Source: CAD feature listing. Evaluate the final solid. Frame: model axes, mm. Face numbers are marked on the shaded views. A direction names the side the tool comes from. Round coordinates to 2 decimals unless told otherwise and drop trailing zeros. Loops run counter-clockwise (first coordinate to the right, second up) from the corner with the lowest first, then second, coordinate; pieces in that order, holes last. Notation, with made-up numbers: (61, 25.25) -> (101, 25.25) arc R24 ccw to (101, 36.25) -> close; hole circle Ø9 at (-26.75, -5). An arc over 180 degrees is marked (long way). Put each result on its own line as item: value. Start each with the question number.
1. Cut plane C-C (x = 3.5). Return the cut outline in (y, z) (1 decimal).
2. Set-up query: the marked faces 1 and 2. Return all of +Z, -Z, +X, -X, +Y, -Y with unobstructed straight access to the full face (end or side cutting, diameter ignored); none if empty.
3. Contact query for flat-ended pins moving along their axis: pin 1 (5 mm diameter, centred on y = 9, z = 25.5, fed in from +X); pin 2 (6.5 mm diameter, centred on y = 8, z = 102, fed in from -X); pin 3 (4 mm diameter, centred on x = 2.5, y = 9, fed in from +Z). Output: stop coordinate, or through.
4. Material intervals for L1, parallel to Y at x = 31.25, z = 58.42; L2, parallel to Z at x = 34, y = 11.75; L3, parallel to X at y = 12, z = 33, sorted ascending.
5. Cut plane A-A (z = 58.42). Return the cut outline in (x, y), then the cut area to 3 significant figures.
6. Cut plane B-B (y = 7.5). Return the cut outline in (x, z), then the cut area to 3 significant figures.
7. Cut plane D-D (y = 12.75). Return the cut outline in (x, z), then the cut area to 3 significant figures.
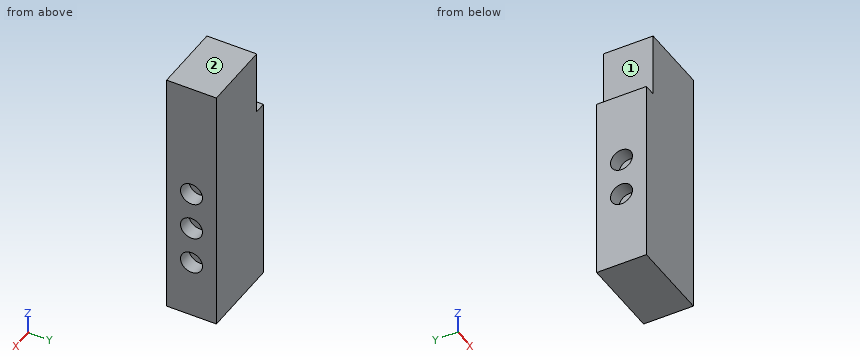
```python
from build123d import *

# Parameters (mm, degrees)
SKETCH1_W           = 35.56
SKETCH1_H           = 21.59
BOSS_EXTRUDE1_DEPTH = 81.28
SKETCH2_W           = 30.48
SKETCH2_H           = 21.59
BOSS_EXTRUDE2_DEPTH = 27.94
SKETCH3_R           = 4.7625
CUT_EXTRUDE1_DEPTH  = 6.35
SKETCH4_R           = 4.7625
CUT_EXTRUDE2_DEPTH  = 6.35


with BuildPart() as part:
    # Sketch1 → Boss-Extrude1 (new body)
    with BuildSketch(Plane.XY):
        with Locations((17.78, 10.795)):
            Rectangle(SKETCH1_W, SKETCH1_H)
    extrude(amount=BOSS_EXTRUDE1_DEPTH)

    # Sketch2 → Boss-Extrude2 (add)
    with BuildSketch(Plane.XY.offset(81.28)):
        with Locations((20.32, 10.795)):
            Rectangle(SKETCH2_W, SKETCH2_H)
    extrude(amount=BOSS_EXTRUDE2_DEPTH)

    # Sketch3 → Cut-Extrude1 (cut)
    with BuildSketch(Plane(origin=(35.56, 0, 0), x_dir=(0, 0, -1), z_dir=(1, 0, 0))):
        with Locations((-25.4, 10.795)):
            Circle(SKETCH3_R)
        with Locations((-41.91, 10.795)):
            Circle(SKETCH3_R)
        with Locations((-58.42, 10.795)):
            Circle(SKETCH3_R)
    extrude(amount=-CUT_EXTRUDE1_DEPTH, mode=Mode.SUBTRACT)

    # Sketch4 → Cut-Extrude2 (cut)
    with BuildSketch(Plane.ZY):
        with Locations((33.655, 10.795)):
            Circle(SKETCH4_R)
        with Locations((50.165, 10.795)):
            Circle(SKETCH4_R)
    extrude(amount=-CUT_EXTRUDE2_DEPTH, mode=Mode.SUBTRACT)


solid = part.part
```
Solution:
1. outline: (0, 0) -> (21.6, 0) -> (21.6, 81.3) -> (0, 81.3) -> close; hole circle Ø9.5 at (10.8, 33.7); hole circle Ø9.5 at (10.8, 50.2)
2. face 1: +Z, -X, +Y, -Y
2. face 2: +Z, +X, -X, +Y, -Y
3. pin 1: stops at x = 29.21
3. pin 2: stops at x = 5.08
3. pin 3: stops at z = 81.28
4. L1: y = 0 to 6.03, 15.56 to 21.59
4. L2: z = 0 to 20.73, 30.07 to 37.24, 46.58 to 53.75, 63.09 to 109.22
4. L3: x = 6.35 to 35.56
5. outline: (0, 0) -> (35.56, 0) -> (35.56, 6.03) -> (29.21, 6.03) -> (29.21, 15.56) -> (35.56, 15.56) -> (35.56, 21.59) -> (0, 21.59) -> close
5. area: 707 mm^2
6. outline: (0, 0) -> (35.56, 0) -> (35.56, 21.96) -> (29.21, 21.96) -> (29.21, 28.84) -> (35.56, 28.84) -> (35.56, 38.47) -> (29.21, 38.47) -> (29.21, 45.35) -> (35.56, 45.35) -> (35.56, 54.98) -> (29.21, 54.98) -> (29.21, 61.86) -> (35.56, 61.86) -> (35.56, 109.22) -> (5.08, 109.22) -> (5.08, 81.28) -> (0, 81.28) -> (0, 53.6) -> (6.35, 53.6) -> (6.35, 46.73) -> (0, 46.73) -> (0, 37.09) -> (6.35, 37.09) -> (6.35, 30.22) -> (0, 30.22) -> close
6. area: 3,520 mm^2
7. outline: (0, 0) -> (35.56, 0) -> (35.56, 21.06) -> (29.21, 21.06) -> (29.21, 29.74) -> (35.56, 29.74) -> (35.56, 37.57) -> (29.21, 37.57) -> (29.21, 46.25) -> (35.56, 46.25) -> (35.56, 54.08) -> (29.21, 54.08) -> (29.21, 62.76) -> (35.56, 62.76) -> (35.56, 109.22) -> (5.08, 109.22) -> (5.08, 81.28) -> (0, 81.28) -> (0, 54.51) -> (6.35, 54.51) -> (6.35, 45.82) -> (0, 45.82) -> (0, 38) -> (6.35, 38) -> (6.35, 29.31) -> (0, 29.31) -> close
7. area: 3,470 mm^2
